```python
from build123d import *

# Parameters (mm, degrees)
IZIM1_R                     = 4.45
Y_KSEKLIK_EKSTR_ZYON1_DEPTH = 5.6
IZIM2_R                     = 10.45
IZIM2_R_2                   = 0.75
Y_KSEKLIK_EKSTR_ZYON2_DEPTH = 2.3
IZIM3_R                     = 2.95
KES_EKSTR_ZYON1_DEPTH       = 1.05
IZIM4_R                     = 4.65
IZIM4_R_2                   = 3.35
KES_EKSTR_ZYON2_DEPTH       = 1.05
IZIM5_R                     = 1.5
KES_EKSTR_ZYON3_DEPTH       = 11.05
IZIM6_R                     = 2.68
KES_EKSTR_ZYON4_DEPTH       = 3.5
KES_EKSTR_ZYON5_DEPTH       = 3.5
DAIRESEL_KAPLAMA1_COUNT     = 24


with BuildPart() as part:
    # Çizim1 → Yükseklik-Ekstrüzyon1 (new body)
    with BuildSketch(Plane.XY):
        Circle(IZIM1_R)
    extrude(amount=Y_KSEKLIK_EKSTR_ZYON1_DEPTH)

    # Çizim2 → Yükseklik-Ekstrüzyon2 (add)
    with BuildSketch(Plane.XY.offset(5.6)):
        Circle(IZIM2_R)
        with Locations((-7.7, 3.4)):
            Circle(IZIM2_R_2, mode=Mode.SUBTRACT)
        with Locations((-7.7, 0)):
            Circle(IZIM2_R_2, mode=Mode.SUBTRACT)
        with Locations((-7.7, -3.4)):
            Circle(IZIM2_R_2, mode=Mode.SUBTRACT)
        with Locations((0, 7.07)):
            Circle(IZIM2_R_2, mode=Mode.SUBTRACT)
        with Locations((3.4, 7.07)):
            Circle(IZIM2_R_2, mode=Mode.SUBTRACT)
        with Locations((-3.4, 7.07)):
            Circle(IZIM2_R_2, mode=Mode.SUBTRACT)
        with Locations(Location((-3.4, -7.07, 0), (0, 0, 180))):
            Circle(IZIM2_R_2, mode=Mode.SUBTRACT)
        with Locations(Location((3.4, -7.07, 0), (0, 0, 180))):
            Circle(IZIM2_R_2, mode=Mode.SUBTRACT)
        with Locations(Location((0, -7.07, 0), (0, 0, 180))):
            Circle(IZIM2_R_2, mode=Mode.SUBTRACT)
        with Locations(Location((7.7, -3.4, 0), (0, 0, 180))):
            Circle(IZIM2_R_2, mode=Mode.SUBTRACT)
        with Locations(Location((7.7, 0, 0), (0, 0, 180))):
            Circle(IZIM2_R_2, mode=Mode.SUBTRACT)
        with Locations(Location((7.7, 3.4, 0), (0, 0, 180))):
            Circle(IZIM2_R_2, mode=Mode.SUBTRACT)
    extrude(amount=-Y_KSEKLIK_EKSTR_ZYON2_DEPTH)

    # Çizim3 → Kes-Ekstrüzyon1 (cut)
    with BuildSketch(Plane.XY.offset(5.6)):
        Circle(IZIM3_R)
    extrude(amount=-KES_EKSTR_ZYON1_DEPTH, mode=Mode.SUBTRACT)

    # Çizim4 → Kes-Ekstrüzyon2 (cut)
    with BuildSketch(Plane.XY.offset(5.6)):
        Circle(IZIM4_R)
        Circle(IZIM4_R_2, mode=Mode.SUBTRACT)
    extrude(amount=-KES_EKSTR_ZYON2_DEPTH, mode=Mode.SUBTRACT)

    # Çizim5 → Kes-Ekstrüzyon3 (cut)
    with BuildSketch(Plane.XY.offset(4.55)):
        Circle(IZIM5_R)
    extrude(amount=-KES_EKSTR_ZYON3_DEPTH, mode=Mode.SUBTRACT)

    # Çizim6 → Kes-Ekstrüzyon4 (cut)
    with BuildSketch(Plane(origin=(0, 0, 0), x_dir=(-1, 0, 0), z_dir=(0, 0, -1))):
        Circle(IZIM6_R)
    extrude(amount=-KES_EKSTR_ZYON4_DEPTH, mode=Mode.SUBTRACT)

    # Çizim7 → Kes-Ekstrüzyon5 (cut)
    with BuildSketch(Plane(origin=(0, 0, 3.5), x_dir=(-1, 0, 0), z_dir=(0, 0, -1))):
        with BuildLine():
            Line((-2.485339529, 1.767933095), (-2.601102839, 1.592722205))
            Line((-2.601102839, 1.592722205), (-2.368659359, 1.253735555))
            ThreePointArc((-2.368659359, 1.253735555), (-2.236024692, 1.477360341), (-2.082344793, 1.687080366))
            Line((-2.082344793, 1.687080366), (-2.485339529, 1.767933095))
        make_face()
    kes_ekstr_zyon5 = extrude(amount=KES_EKSTR_ZYON5_DEPTH, mode=Mode.SUBTRACT)

    # Dairesel Kaplama1: Kes-Ekstrüzyon5 ×24 about axis
    dairesel_kaplama1_axis = Axis((0, 0, 0), (0, 0, 1))
    for i in range(1, DAIRESEL_KAPLAMA1_COUNT):
        add(kes_ekstr_zyon5.rotate(dairesel_kaplama1_axis, i * 360 / DAIRESEL_KAPLAMA1_COUNT), mode=Mode.SUBTRACT)


solid = part.part
```
Can you work these out from the model? Positions are in its coordinate system, mm. A direction names the side the tool comes from. Coordinates: 2 decimals unless noted, no trailing zeros. Loops run counter-clockwise (first coordinate to the right, second up) from the corner with the lowest first, then second, coordinate; pieces in that order, holes last.
1) I need wall thicknesses on probe 1 along Y at (x, z) = (0, 4.15); probe 2 along Y at (x, z) = (0, 4.9); probe 3 along X at (y, z) = (6.5, 3.45). Which ranges of each line are inside material? Lowest first, please.
2) Which directions (+Z, -Z, +X, -X, +Y, -Y) give clear straight access to the entire face, cutting with the end or side of a thin tool? Please do faces 1 (the cylindrical face through (2.65, 7.1, 4.47)), 2 (the cylindrical face through (-3.347, 0.147, 5.082)), 3 (the flat face through (4.5, -2.2, 3.3)).
3) For pin 1 (2.5 mm diameter, centred on x = 7.7, y = -3.4, fed in from -Z); pin 2 (1 mm diameter, centred on x = -2, z = 1, fed in from -Y); pin 3 (0.9 mm diameter, centred on x = 7.7, y = 0, fed in from -Z); pin 4 (2 mm diameter, centred on x = 4, z = 4, fed in from +Y), each with a flat end and sliding along its axis, tell me the tip position at first contact or that it passes through.
4) Imagine slicing it at A-A on x = -7.5. List the corners of the cut face in (y, z) for me, plus the area to 3 significant figures.
5) Imagine slicing it at B-B on z = 4.2. State how many separate pieces and enclosed holes the cut face has, plus the area to 3 significant figures.
6) Imagine slicing it at D-D on x = 5.75. List the corners of the cut face in (y, z) for me.
7) Imagine slicing it at C-C on y = 7.07. List the corners of the cut face in (x, z) for me, plus the area to 3 significant figures.
8) Thinking about a two-plate mould opening in X: for faces 4 (the cylindrical face through (-7.702, 7.063, 4.466)), 5 (the cylindrical face through (-8.25, 3.91, 4.47)), 6 (the flat face through (1, -3, 5.6)), which applies, pulls with the +X half, pulls with the -X half, needs draft (parallel to the pull), parting line crosses it, or undercut?
Completed:
1. probe 1: y = -10.45 to -7.82, -6.32 to -1.5, 1.5 to 6.32, 7.82 to 10.45
1. probe 2: y = -10.45 to -7.82, -6.32 to -4.65, -3.35 to -2.95, 2.95 to 3.35, 4.65 to 6.32, 7.82 to 10.45
1. probe 3: x = -8.18 to -3.89, -2.91 to -0.49, 0.49 to 2.91, 3.89 to 8.18
2. face 1: +Z, -Z
2. face 2: +Z
2. face 3: -Z
3. pin 1: stops at z = 3.3
3. pin 2: stops at y = -4.19
3. pin 3: passes through
3. pin 4: stops at y = 10.01
4. outline: (-7.28, 3.3) - (-4.12, 3.3) - (-4.12, 5.6) - (-7.28, 5.6) - close; (-2.68, 3.3) - (-0.72, 3.3) - (-0.72, 5.6) - (-2.68, 5.6) - close; (0.72, 3.3) - (2.68, 3.3) - (2.68, 5.6) - (0.72, 5.6) - close; (4.12, 3.3) - (7.28, 3.3) - (7.28, 5.6) - (4.12, 5.6) - close
4. area: 23.5 mm2
5. separate pieces: 1
5. enclosed holes: 13
5. area: 315 mm2
6. outline: (-8.73, 3.3) - (8.73, 3.3) - (8.73, 5.6) - (-8.73, 5.6) - close
7. outline: (-7.7, 3.3) - (-4.15, 3.3) - (-4.15, 5.6) - (-7.7, 5.6) - close; (-2.65, 3.3) - (-0.75, 3.3) - (-0.75, 5.6) - (-2.65, 5.6) - close; (0.75, 3.3) - (2.65, 3.3) - (2.65, 5.6) - (0.75, 5.6) - close; (4.15, 3.3) - (7.7, 3.3) - (7.7, 5.6) - (4.15, 5.6) - close
7. area: 25.0 mm2
8. face 4: parting line crosses it
8. face 5: undercut
8. face 6: needs draft
